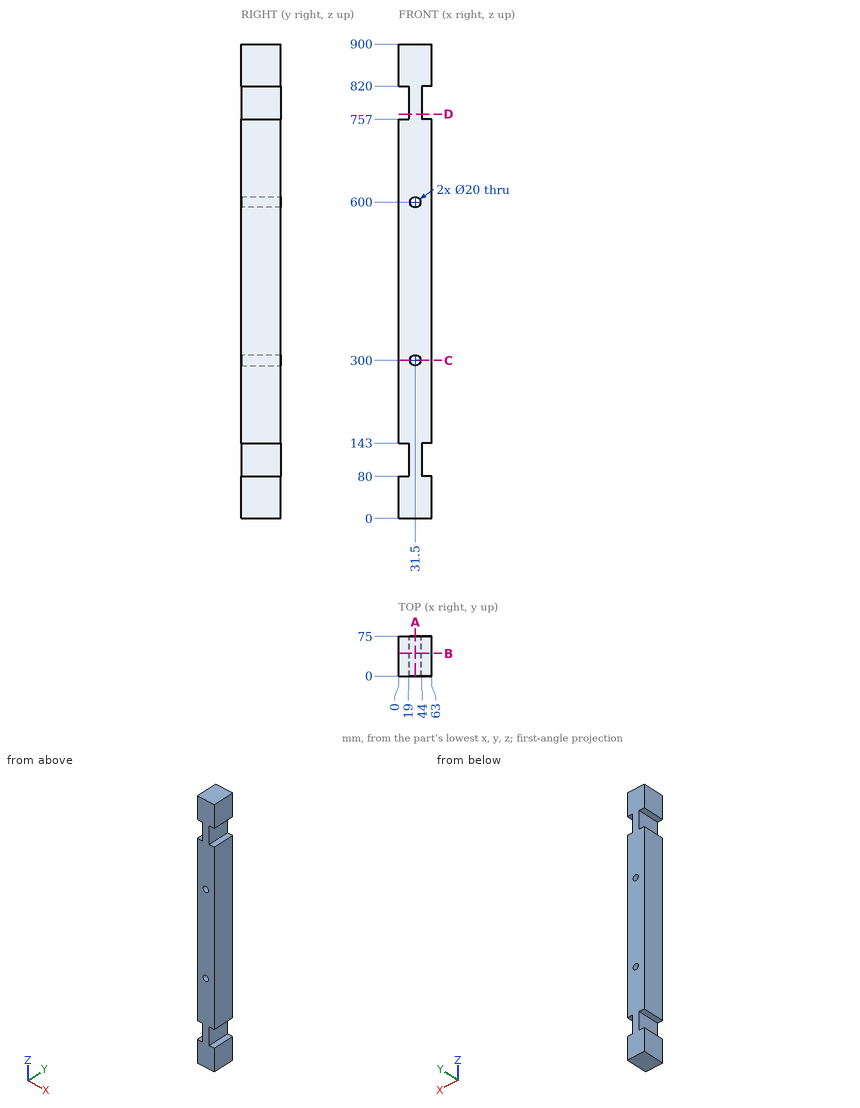
Here's the drawing with two shaded views (mm, measured from the low corner). I have some questions. Coordinates: 2 decimals unless noted, no trailing zeros. Order: outer loops, then holes, each group sorted by start corner. A loop starts at its lowest first (then second) coordinate and runs counter-clockwise, first axis right, second up.
Q1. Suppose I cut it at C-C on z = 300. Please give me the cut outline in (x, y).
Q2. Please list where these lines run through material, in increasing order: L1, parallel to Z at x = 5, y = 58; L2, parallel to Z at x = 31, y = 58; L3, parallel to X at y = 56, z = 600.
Q3. Suppose I cut it at A-A on x = 31.5. Please give me the cut outline in (y, z).
Q4. Suppose I cut it at D-D on z = 767. Please give me the cut outline in (x, y).
Q5. Suppose I cut it at B-B on y = 43. Please give me the cut outline in (x, z).
Q6. Will these pins go through, and if not, where does the flat tip stop? pin 1 (12 mm diameter, centred on y = 37, z = 101.5, fed in from -X); pin 2 (19 mm diameter, centred on y = 28, z = 783.5, fed in from +X).
Answer:
1. outline: (0, 0) - (21.5, 0) - (21.5, 75) - (0, 75) - close; (41.5, 0) - (63, 0) - (63, 75) - (41.5, 75) - close
2. L1: z = 0 to 80, 143 to 757, 820 to 900
2. L2: z = 0 to 290.01, 309.99 to 590.01, 609.99 to 900
2. L3: x = 0 to 21.5, 41.5 to 63
3. outline: (0, 0) - (75, 0) - (75, 290) - (0, 290) - close; (0, 310) - (75, 310) - (75, 590) - (0, 590) - close; (0, 610) - (75, 610) - (75, 900) - (0, 900) - close
4. outline: (19, 0) - (44, 0) - (44, 75) - (19, 75) - close
5. outline: (0, 0) - (63, 0) - (63, 80) - (44, 80) - (44, 143) - (63, 143) - (63, 757) - (44, 757) - (44, 820) - (63, 820) - (63, 900) - (0, 900) - (0, 820) - (19, 820) - (19, 757) - (0, 757) - (0, 143) - (19, 143) - (19, 80) - (0, 80) - close; hole circle Ø20 at (31.5, 300); hole circle Ø20 at (31.5, 600)
6. pin 1: stops at x = 19
6. pin 2: stops at x = 44
